Read the model definition and answer for the solid it produces. Units are mm, in the model's axes. Give positions to 0.01 mm unless a question says otherwise; leave off trailing zeros. Order: outer loops, then holes, each group sorted by start corner. A loop starts at its lowest first (then second) coordinate and runs counter-clockwise, first axis right, second up. Notation, with made-up numbers: M 9,-38 L 17,-38 A21 cw 17,-13 Z; hole C 82,-3.5 d7. An arc over 180 degrees is marked long. Write item = value, one per line. Start each with the question number.
from build123d import *

# Parameters (mm, degrees)
F0_R     = 25.4
F1_DEPTH = 444.5
F2_R     = 22.225
F3_DEPTH = 431.8
F4_R     = 25.4
F5_DEPTH = 12.7
F6_R     = 5.08
F7_R     = 5.08


with BuildPart() as f1:
    # F0 (on Top) → F1 (new body)
    with BuildSketch(Plane.XY):
        Circle(F0_R)
    extrude(amount=F1_DEPTH)

    # F2 (on face) → F3 (cut)
    with BuildSketch(Plane.XY.offset(444.5)):
        Circle(F2_R)
    extrude(amount=-F3_DEPTH, mode=Mode.SUBTRACT)

    # F4 (on face) → F5 (join)
    with BuildSketch(Plane.XY.offset(444.5)):
        Circle(F4_R)
    extrude(amount=F5_DEPTH)

    # F6
    f6_edges = [f1.edges().sort_by_distance(p)[0] for p in [
        (-25.4, 0, 457.2),
    ]]
    fillet(f6_edges, radius=F6_R)

    # F7
    f7_edges = [f1.edges().sort_by_distance(p)[0] for p in [
        (-25.4, 0, 0),
    ]]
    fillet(f7_edges, radius=F7_R)


solid = f1.part
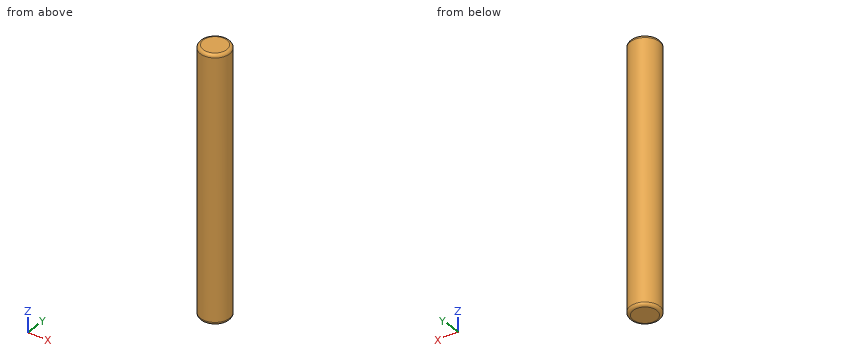
1) Find the intervals of material crossed by probe 1 along Y at (x, z) = (0, 300) (3 decimals); probe 2 along Z at (x, y) = (-16, -4); probe 3 along X at (y, z) = (-1, 318.5), in increasing order. Write a range as [from, to].
2) Find section C-C on z = 182.5. Determine the outline of the cut face in (x, y) (3 decimals), plus the area to 3 significant figures.
3) Each of these flat-tipped pins is pushed along its axis until it touches: P1, Ø4, axis at y = -12.5, z = 207, coming from the -X side; P2, Ø10, axis at y = -6.5, z = 157.5, coming from the -X side; P3, Ø1.5, axis at x = 11, z = 231, coming from the +Y side. Where does it stop, or does it pass through?
4) Find section A-A on y = 0. Determine the outline of the cut face in (x, z) (3 decimals).
Numbers:
q1.probe_1 = [-25.4, -22.225], [22.225, 25.4]
q1.probe_2 = [0, 12.7], [444.5, 457.2]
q1.probe_3 = [-25.38, -22.2], [22.2, 25.38]
q2.outline = C 0,0 d50.8; hole C 0,0 d44.45
q2.area = 475 mm2
q3.P1 = -23.13
q3.P2 = -25.36
q3.P3 = 23.24
q4.outline = M -25.4,5.08 A5.08 ccw -20.32,0 L 20.32,0 A5.08 ccw 25.4,5.08 L 25.4,452.12 A5.08 ccw 20.32,457.2 L -20.32,457.2 A5.08 ccw -25.4,452.12 Z; hole M -22.225,12.7 L 22.225,12.7 L 22.225,444.5 L -22.225,444.5 Z
